Here's how the part is built. I have some questions about the finished solid (model axes, mm). Face numbers are marked on the shaded views. A direction names the side the tool comes from. Coordinates: 2 decimals unless noted, no trailing zeros. Write each loop counter-clockwise with the first axis right and the second up, starting at its lowest first coordinate (ties: lowest second). Pieces come first, ordered by that corner, then holes. Notation, with made-up numbers: (44.5, 83) -> (101.5, 83) arc R21 cw to (101.5, 104) -> close; hole circle Ø8 at (-15.5, 41.25). An arc over 180 degrees is marked (long way). Answer in a Markdown table with one row per item. Add a question column.
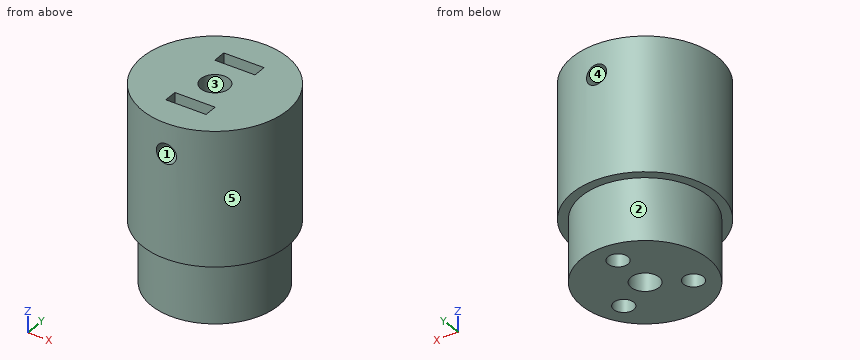
from build123d import *

# Parameters (mm, degrees)
SKETCH1_R           = 9.5
SKETCH1_R_2         = 2.1
BOSS_EXTRUDE1_DEPTH = 9.26
SKETCH2_R           = 10.85
SKETCH2_R_2         = 2.1
BOSS_EXTRUDE2_DEPTH = 20
SKETCH3_W           = 6
SKETCH3_H           = 2
CUT_EXTRUDE1_DEPTH  = 12
SKETCH4_R           = 1.5
CUT_EXTRUDE2_DEPTH  = 39.01
SKETCH5_R           = 1.5
CUT_EXTRUDE3_DEPTH  = 12


with BuildPart() as part:
    # Sketch1 → Boss-Extrude1 (new body)
    with BuildSketch(Plane.XY):
        Circle(SKETCH1_R)
        Circle(SKETCH1_R_2, mode=Mode.SUBTRACT)
    extrude(amount=BOSS_EXTRUDE1_DEPTH)

    # Sketch2 → Boss-Extrude2 (add)
    with BuildSketch(Plane.XY.offset(9.26)):
        Circle(SKETCH2_R)
        Circle(SKETCH2_R_2, mode=Mode.SUBTRACT)
    extrude(amount=BOSS_EXTRUDE2_DEPTH)

    # Sketch3 → Cut-Extrude1 (cut)
    with BuildSketch(Plane.XY.offset(29.26)):
        with Locations((0, 5.422033923)):
            Rectangle(SKETCH3_W, SKETCH3_H)
        with Locations((0, -5.422033923)):
            Rectangle(SKETCH3_W, SKETCH3_H)
    extrude(amount=-CUT_EXTRUDE1_DEPTH, mode=Mode.SUBTRACT)

    # Sketch4 → Cut-Extrude2 (cut, through all)
    with BuildSketch(Plane(origin=(0, 10.85, 0), x_dir=(1, 0, 0), z_dir=(0, 1, 0))):
        with Locations(Location((0, -24.76, 0), (0, 0, 180))):
            Circle(SKETCH4_R)
    extrude(amount=-CUT_EXTRUDE2_DEPTH, mode=Mode.SUBTRACT)

    # Sketch5 → Cut-Extrude3 (cut)
    with BuildSketch(Plane(origin=(0, 0, 0), x_dir=(-1, 0, 0), z_dir=(0, 0, -1))):
        with Locations((0, 6)):
            Circle(SKETCH5_R)
        with Locations((5.196152423, -3)):
            Circle(SKETCH5_R)
        with Locations((-5.196152423, -3)):
            Circle(SKETCH5_R)
    extrude(amount=-CUT_EXTRUDE3_DEPTH, mode=Mode.SUBTRACT)


solid = part.part
Q1. Imagine slicing it at D-D on y = -8.5. Please give me the cut outline in (x, z).
Q2. Imagine slicing it at A-A on y = 0. Please give me the cut outline in (x, z), plus the area to 3 significant figures.
Q3. For the marked faces 1 and 2, which set-ups out of +Z, -Z, +X, -X, +Y, -Y let a thin tool reach every point of the face, with its end or its side?
Q4. Imagine slicing it at C-C on z = 2.25. Please give me the cut outline in (x, y).
Q5. I need wall thicknesses on line 1 (Z direction, x = 0, y = 7.4); line 2 (Z direction, x = 0, y = -2.35); line 3 (X direction, y = -5.25, z = 28). Which ranges of each line are inside material? Lowest first, please. Write a range as [from, to].
Q6. Imagine slicing it at B-B on z = 22.5. Please give me the cut outline in (x, y).
Q7. I'm going to push flat-ended pins straight in: P1, Ø0.6, axis at y = 5.5, z = 21.5, coming from the +X side; P2, Ø2.5, axis at x = 0, z = 24.76, coming from the +Y side; P3, Ø1.6, axis at y = -5, z = 26, coming from the +X side; P4, Ø10, axis at x = 6, z = 20.5, coming from the -Y side. Where does each tip first touch, or does it pass through?
Q8. If we mould it in two halves opening along Y, with no side actions, what happens to the marked faces 3, 4 and 5? For each: pulls with the +Y half, pulls with the -Y half, needs draft (parallel to the pull), parting line crosses it, or undercut.
Result sheet:
| question | item | result |
|---|---|---|
| 1 | outline | (-6.74, 9.26) -> (-4.24, 9.26) -> (-4.24, 0) -> (4.24, 0) -> (4.24, 9.26) -> (6.74, 9.26) -> (6.74, 29.26) -> (-6.74, 29.26) -> close; hole circle Ø3 at (0, 24.76) |
| 2 | outline | (-10.85, 9.26) -> (-9.5, 9.26) -> (-9.5, 0) -> (-2.1, 0) -> (-2.1, 29.26) -> (-10.85, 29.26) -> close; (2.1, 0) -> (9.5, 0) -> (9.5, 9.26) -> (10.85, 9.26) -> (10.85, 29.26) -> (2.1, 29.26) -> close |
| 2 | area | 487 mm^2 |
| 3 | face 1 | +Y, -Y |
| 3 | face 2 | -Z |
| 4 | outline | circle Ø19 at (0, 0); hole circle Ø3 at (-5.2, -3); hole circle Ø4.2 at (0, 0); hole circle Ø3 at (0, 6); hole circle Ø3 at (5.2, -3) |
| 5 | line 1 | z = [12, 23.26], [26.26, 29.26] |
| 5 | line 2 | z = [0, 23.26], [26.26, 29.26] |
| 5 | line 3 | x = [-9.5, -3], [3, 9.5] |
| 6 | outline | circle Ø21.7 at (0, 0); hole (-3, -6.42) -> (3, -6.42) -> (3, -4.42) -> (-3, -4.42) -> close; hole (-3, 4.42) -> (3, 4.42) -> (3, 6.42) -> (-3, 6.42) -> close; hole circle Ø4.2 at (0, 0) |
| 7 | P1 | stops at x = 9.52 |
| 7 | P2 | passes through |
| 7 | P3 | stops at x = 10 |
| 7 | P4 | stops at y = -10.8 |
| 8 | face 3 | undercut |
| 8 | face 4 | needs draft |
| 8 | face 5 | parting line crosses it |
